Can you work these out from the model? Positions are in its coordinate system, mm. Face numbers are marked on the shaded views. A direction names the side the tool comes from. Give positions to 0.01 mm unless a question says otherwise; leave off trailing zeros. Write each loop counter-clockwise with the first axis right and the second up, starting at its lowest first coordinate (ties: lowest second). Pieces come first, ordered by that corner, then holes. Notation, with made-up numbers: M 29,-25.5 L 64,-25.5 A30 ccw 64,7.5 Z; hole C 77,8.5 d9. An arc over 180 degrees is marked long. Use CSV: the item, a comma, the result in double quotes. Start each with the question number.
from build123d import *

# Parameters (mm, degrees)
SKETCH9_R          = 1.25
CUT_EXTRUDE2_DEPTH = 26.5
SKETCH13_W         = 1.25
SKETCH13_H         = 11


with BuildPart() as part:
    # Sketch11 → Revolve1 (revolve)
    with BuildSketch(Plane.XY):
        Polygon((2.5, 25.5), (11, 25.5), (11, 25), (9, 23), (9, 6), (11, 4), (11, 0), (2.5, 0), align=None)
    revolve(axis=Axis((0, 0, 0), (0, 1, 0)))

    # Sketch9 → Cut-Extrude2 (cut, through all)
    with BuildSketch(Plane.XZ):
        with Locations((5.152851153, -2.975)):
            Circle(SKETCH9_R)
    extrude(amount=-CUT_EXTRUDE2_DEPTH, mode=Mode.SUBTRACT)

    # Sketch10 → Cut-Revolve1 (revolve, cut)
    with BuildSketch(Plane.XY):
        Polygon((5.095658377, -0.530330086), (4.565328291, 0), (9.782664146, 5.217335854), (10.312994231, 4.687005769), align=None)
    revolve(axis=Axis((10.312994231, 4.687005769, 0), (-0.707106781, -0.707106781, 0)), mode=Mode.SUBTRACT)

    # Sketch10_3 → Cut-Revolve2 (revolve, cut)
    with BuildSketch(Plane.XY):
        Polygon((10.41573594, 22.407308798), (6.792714652, 26.030330086), (6.262384566, 25.5), (9.885405854, 21.876978712), align=None)
    revolve(axis=Axis((10.41573594, 22.407308798, 0), (-0.707106781, 0.707106781, 0)), mode=Mode.SUBTRACT)

    # Sketch13 → M3x0.5 Tapped Hole1 (revolve, cut)
    with BuildSketch(Plane(origin=(0, 2, 0), x_dir=(0, 0, -1), z_dir=(0, 1, 0))):
        with Locations((0.625, 5.5)):
            Rectangle(SKETCH13_W, SKETCH13_H)
    revolve(axis=Axis((6.35, 2, 0), (-1, 0, 0)), mode=Mode.SUBTRACT)


solid = part.part
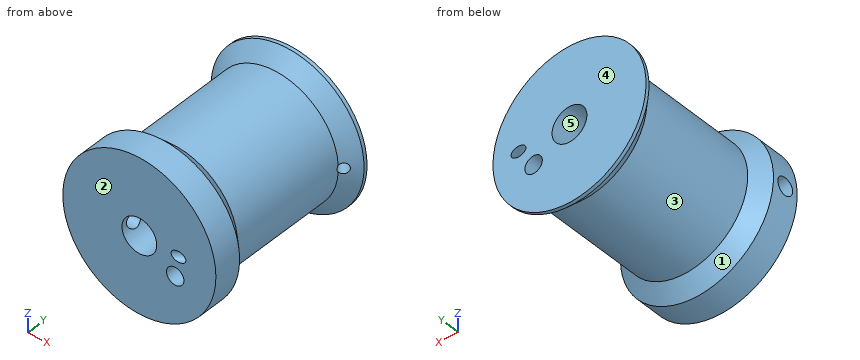
(1) Will these pins go through, and if not, where does the flat tip stop? pin 1 Ø2 at (y, z) = (11, -0.5) entering from +X; pin 2 Ø4 at (x, y) = (-7.5, 8) entering from -Z; pin 3 Ø1.5 at (y, z) = (5.5, 2.5) entering from +X.
(2) I want a section at B-B (x = 0). Write out the boundary of the cut face in (y, z).
(3) I want a section at D-D (y = 2). State how many separate pieces and enclosed holes the cut face has, and give its area (3 significant figures).
(4) I want a section at C-C (y = 13.5). Write out the boundary of the cut face in (x, z) (3 decimals), and give its area (3 significant figures).
(5) Thinking about a two-plate mould opening in X: for the marked faces 3, 4 and 5, which applies, released by +X, released by -X, zero draft, split by the parting line, or undercut?
(6) Please list where these lines run through material, in increasing order: L1, parallel to Y at x = -4.5, z = 0; L2, parallel to X at y = 16, z = 0; L3, parallel to Y at x = 5.5, z = -8.5. Write a range as [from, to].
(7) I want a section at A-A (z = 0). Write out the boundary of the cut face in (x, y).
(8) Which directions (+Z, -Z, +X, -X, +Y, -Y) give clear straight access to the entire face, cutting with the end or side of a thin tool? Please do the marked faces 1 and 2.
Geometry results:
1,pin 1,"stops at x = 9"
1,pin 2,"stops at z = -7.12"
1,pin 3,"stops at x = 9.96"
2,outline,"M 0,-11 L 4,-11 L 6,-9 L 23,-9 L 25,-11 L 25.5,-11 L 25.5,-2.5 L 0,-2.5 Z; M 0,2.5 L 25.5,2.5 L 25.5,11 L 25,11 L 23,9 L 6,9 L 4,11 L 0,11 Z"
3,separate pieces,"1"
3,enclosed holes,"2"
3,area,"332 mm2"
4,outline,"C 0,0 d18; hole C 0,0 d5; hole C 5.153,-2.975 d2.5"
4,area,"230 mm2"
5,face 3,"split by the parting line"
5,face 4,"zero draft"
5,face 5,"undercut"
6,L1,"y = [0, 0.75], [3.25, 25.5]"
6,L2,"x = [-9, -2.5], [2.5, 9]"
6,L3,"y = [0, 4.88], [24.12, 25.5]"
7,outline,"M -11,0 L -2.5,0 L -2.5,0.75 L -11,0.75 Z; M -11,3.25 L -2.5,3.25 L -2.5,25.5 L -11,25.5 L -11,25 L -9,23 L -9,6 L -11,4 Z; M 2.5,0 L 4.57,0 L 9.78,5.22 L 9,6 L 9,22.76 L 6.26,25.5 L 2.5,25.5 Z; M 6.69,0 L 11,0 L 11,4 L 10.84,4.16 Z; M 8.38,25.5 L 9.94,23.94 L 11,25 L 11,25.5 Z"
8,face 1,"none"
8,face 2,"+Z, -Z, +X, -X, -Y"
